Geometry check sheet. Reference: the model listing, model coordinates, mm. Face numbers are marked on the shaded views. A direction names the side the tool comes from. Give positions to 0.01 mm unless a question says otherwise; leave off trailing zeros. Order: outer loops, then holes, each group sorted by start corner. A loop starts at its lowest first (then second) coordinate and runs counter-clockwise, first axis right, second up.
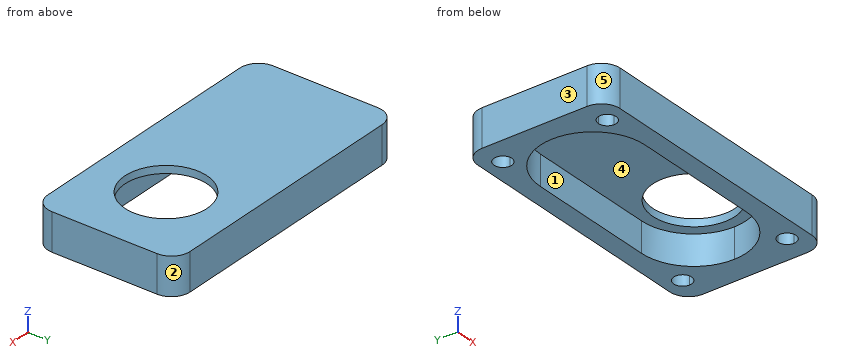
from build123d import *

# Parameters (mm, degrees)
F1_DEPTH = 10
F2_R     = 11
F3_DEPTH = 20
F5_DEPTH = 6
F7_DEPTH = 8


# Not quite as in the source:
# - a feature names something its author has since deleted; it is built from what else it names


with BuildPart() as f1:
    # F0 (on Top) → F1 (new body)
    with BuildSketch(Plane.XY):
        with BuildLine():
            Line((33.1, 19.05), (-33.1, 19.05))
            ThreePointArc((-33.1, 19.05), (-36.6355339059, 17.5855339059), (-38.1, 14.05))
            Line((-38.1, 14.05), (-38.1, -14.05))
            ThreePointArc((-38.1, -14.05), (-36.6355339059, -17.5855339059), (-33.1, -19.05))
            Line((-33.1, -19.05), (33.1, -19.05))
            ThreePointArc((33.1, -19.05), (36.6355339059, -17.5855339059), (38.1, -14.05))
            Line((38.1, -14.05), (38.1, 14.05))
            ThreePointArc((38.1, 14.05), (36.6355339059, 17.5855339059), (33.1, 19.05))
        make_face()
    extrude(amount=F1_DEPTH)

    # F2 (on Top) → F3 (cut)
    with BuildSketch(Plane.XY):
        with Locations((16.8899707496, 0)):
            Circle(F2_R)
    extrude(amount=F3_DEPTH, mode=Mode.SUBTRACT)

    # F4 (on Top) → F5 (cut)
    with BuildSketch(Plane.XY):
        with BuildLine():
            Line((31, -14), (31, -11.625))
            ThreePointArc((31, -11.625), (29.3206213947, -12.3206213947), (28.625, -14))
            Line((28.625, -14), (31, -14))
        make_face()
        with BuildLine():
            ThreePointArc((33.375, -14), (32.6793786053, -12.3206213947), (31, -11.625))
            Line((31, -11.625), (31, -14))
            Line((31, -14), (28.625, -14))
            ThreePointArc((28.625, -14), (31, -16.375), (33.375, -14))
        make_face()
        with BuildLine():
            ThreePointArc((-28.625, -14), (-29.3206213947, -12.3206213947), (-31, -11.625))
            Line((-31, -11.625), (-31, -14))
            Line((-31, -14), (-28.625, -14))
        make_face()
        with BuildLine():
            Line((-31, -14), (-31, -11.625))
            ThreePointArc((-31, -11.625), (-32.6793786053, -15.6793786053), (-28.625, -14))
            Line((-28.625, -14), (-31, -14))
        make_face()
        with BuildLine():
            Line((-31, 14), (-28.625, 14))
            ThreePointArc((-28.625, 14), (-32.6793786053, 15.6793786053), (-31, 11.625))
            Line((-31, 11.625), (-31, 14))
        make_face()
        with BuildLine():
            ThreePointArc((-31, 11.625), (-29.3206213947, 12.3206213947), (-28.625, 14))
            Line((-28.625, 14), (-31, 14))
            Line((-31, 14), (-31, 11.625))
        make_face()
        with BuildLine():
            Line((31, 14), (28.625, 14))
            ThreePointArc((28.625, 14), (29.3206213947, 12.3206213947), (31, 11.625))
            Line((31, 11.625), (31, 14))
        make_face()
        with BuildLine():
            ThreePointArc((33.375, 14), (31, 16.375), (28.625, 14))
            Line((28.625, 14), (31, 14))
            Line((31, 14), (31, 11.625))
            ThreePointArc((31, 11.625), (32.6793786053, 12.3206213947), (33.375, 14))
        make_face()
    extrude(amount=F5_DEPTH, mode=Mode.SUBTRACT)

    # F6 (on Top) → F7 (cut)
    with BuildSketch(Plane.XY):
        with BuildLine():
            Line((16.8287921697, 14), (-18, 14))
            ThreePointArc((-18, 14), (-27.8994949366, 9.8994949366), (-32, 0))
            ThreePointArc((-32, 0), (-27.8994949366, -9.8994949366), (-18, -14))
            Line((-18, -14), (16.8287921697, -14))
            ThreePointArc((16.8287921697, -14), (26.7282871063, -9.8994949366), (30.8287921697, 0))
            ThreePointArc((30.8287921697, 0), (26.7282871063, 9.8994949366), (16.8287921697, 14))
        make_face()
    extrude(amount=F7_DEPTH, mode=Mode.SUBTRACT)


solid = f1.part
Item 1: Sectioned sample at A-A (z = 4.5). Enter the section's corners in (x, y) (3 decimals).
Reported:
outline: (-38.1, -14.05) arc R5 ccw to (-33.1, -19.05) - (33.1, -19.05) arc R5 ccw to (38.1, -14.05) - (38.1, 14.05) arc R5 ccw to (33.1, 19.05) - (-33.1, 19.05) arc R5 ccw to (-38.1, 14.05) - close; hole circle Ø4.75 at (-31, -14); hole circle Ø4.75 at (-31, 14); hole (-18, -14) - (16.829, -14) arc R14 ccw to (16.829, 14) - (-18, 14) arc R14 ccw to start; hole circle Ø4.75 at (31, -14); hole circle Ø4.75 at (31, 14)
Item 2: Sectioned sample at B-B (y = -4.5). Enter the section's corners in (x, z).
Reported:
outline: (-38.1, 0) - (-31.26, 0) - (-31.26, 8) - (6.85, 8) - (6.85, 10) - (-38.1, 10) - close; (26.93, 8) - (30.09, 8) - (30.09, 0) - (38.1, 0) - (38.1, 10) - (26.93, 10) - close
Item 3: Gauge pin test, flat ends, axial feed: pin 1 (1 mm diameter, centred on x = 21.5, y = -9, fed in from -Z); pin 2 (2.5 mm diameter, centred on x = 30.5, y = -13.5, fed in from -Z); pin 3 (8.5 mm diameter, centred on x = -2.5, y = -3.5, fed in from -Z). Record the tip position at first contact, or that the pin passes through.
Reported:
pin 1: passes through
pin 2: stops at z = 6
pin 3: stops at z = 8
Item 4: Set-up check for the marked faces 1 and 2: record each of +Z, -Z, +X, -X, +Y, -Y from which the full face is reachable in a straight line by a thin tool's end or side.
Reported:
face 1: -Z
face 2: +Z, -Z, +X, +Y
Item 5: Sectioned sample at D-D (x = -30). Enter the section's corners in (y, z), and give its area (3 significant figures).
Reported:
outline: (-19.05, 0) - (-16.15, 0) - (-16.15, 6) - (-11.85, 6) - (-11.85, 0) - (-7.21, 0) - (-7.21, 8) - (7.21, 8) - (7.21, 0) - (11.85, 0) - (11.85, 6) - (16.15, 6) - (16.15, 0) - (19.05, 0) - (19.05, 10) - (-19.05, 10) - close
area: 214 mm2
Item 6: Scan lines: L1, parallel to X at y = 0, z = 8.75; L2, parallel to Y at x = 15, z = 1.25; L3, parallel to Z at x = -23.5, y = -12.5. Record each from-to range of solid material in increasing order.
Reported:
L1: x = -38.1 to 5.89, 27.89 to 38.1
L2: y = -19.05 to -14, 14 to 19.05
L3: z = 8 to 10
Item 7: Draft check along Y on the marked faces 3, 4 and 5. Enter one of: released by +Y, released by -Y, zero draft, split by the parting line, or undercut.
Reported:
face 3: zero draft
face 4: undercut
face 5: released by -Y
Item 8: Sectioned sample at C-C (x = 18). Enter the section's corners in (y, z), and give its area (3 significant figures).
Reported:
outline: (-19.05, 0) - (-13.95, 0) - (-13.95, 8) - (-10.94, 8) - (-10.94, 10) - (-19.05, 10) - close; (10.94, 8) - (13.95, 8) - (13.95, 0) - (19.05, 0) - (19.05, 10) - (10.94, 10) - close
area: 114 mm2
